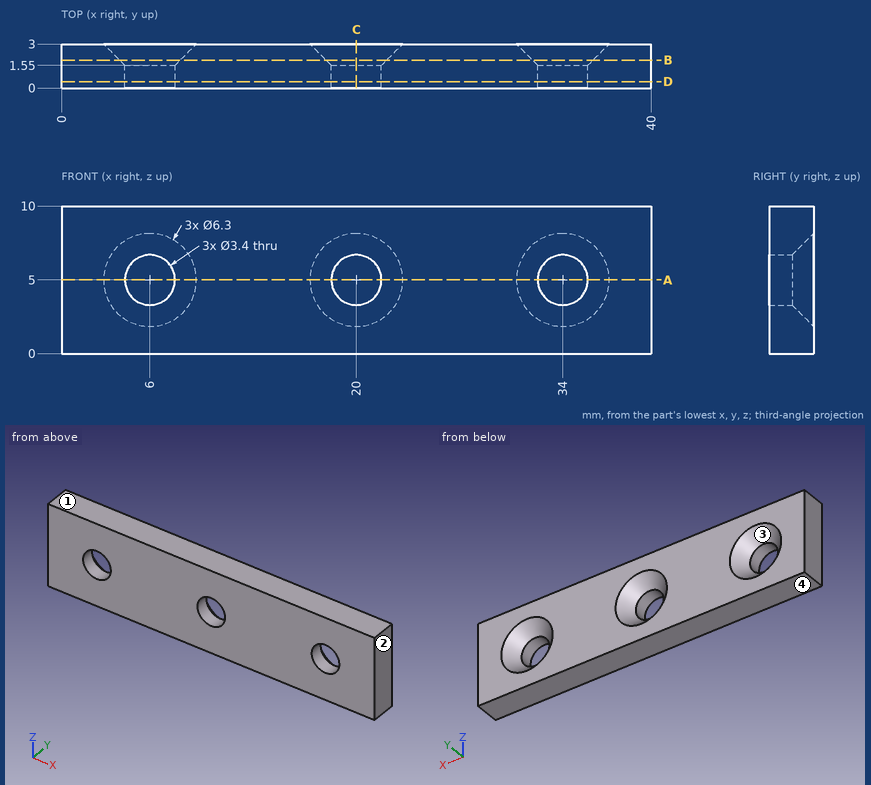
Design review of the part shown in the three views and the two pictorial views. Dimensions are in mm from the part's minimum x, y and z. Give positions to 0.01 mm unless a question says otherwise; leave off trailing zeros. Order: outer loops, then holes, each group sorted by start corner. A loop starts at its lowest first (then second) coordinate and runs counter-clockwise, first axis right, second up. Notation, with made-up numbers: M -37,23 L 10,23 A19 ccw 10,59 Z; hole C -36.75,10.25 d4. An arc over 180 degrees is marked long. Answer in a Markdown table with one row per item. Add a question column.
(1) For pin 1 (4 mm diameter, centred on x = 6, z = 5, fed in from +Y); pin 2 (2.5 mm diameter, centred on x = 34, z = 5, fed in from +Y); pin 3 (3 mm diameter, centred on x = 7.5, z = 5, fed in from +Y), all flat-tipped, find the tip position at first contact; note any pin that passes through.
(2) Consider section D-D on y = 0.45. State the section outline as (x, z) points.
(3) Wall thickness on probe 1 along X at (y, z) = (0.7, 5); probe 2 along Z at (x, y) = (6, 0.8); probe 3 along X at (y, z) = (1.9, 5): over which ranges is each line inside the solid? List them lowest first. Write a range as [from, to].
(4) Mouldability with a two-part tool opening along Z and no side actions: class the marked faces 1, 2, 3 and 4 as +Z half, -Z half, draft (parallel to the pull), parting line (faces both ways), or undercut.
(5) Consider section C-C on x = 20. State the section outline as (y, z) points.
(6) Consider section B-B on y = 1.9. State the section outline as (x, z) points, and give its area (3 significant figures).
(7) Consider section A-A on z = 5. State the section outline as (x, y) points.
Evaluation:
| question | item | result |
|---|---|---|
| 1 | pin 1 | stops at y = 1.85 |
| 1 | pin 2 | passes through |
| 1 | pin 3 | stops at y = 2.85 |
| 2 | outline | M 0,0 L 40,0 L 40,10 L 0,10 Z; hole C 6,5 d3.4; hole C 20,5 d3.4; hole C 34,5 d3.4 |
| 3 | probe 1 | x = [0, 4.3], [7.7, 18.3], [21.7, 32.3], [35.7, 40] |
| 3 | probe 2 | z = [0, 3.3], [6.7, 10] |
| 3 | probe 3 | x = [0, 3.95], [8.05, 17.95], [22.05, 31.95], [36.05, 40] |
| 4 | face 1 | +Z half |
| 4 | face 2 | draft |
| 4 | face 3 | undercut |
| 4 | face 4 | -Z half |
| 5 | outline | M 0,0 L 3,0 L 3,1.85 L 1.55,3.3 L 0,3.3 Z; M 0,6.7 L 1.55,6.7 L 3,8.15 L 3,10 L 0,10 Z |
| 6 | outline | M 0,0 L 40,0 L 40,10 L 0,10 Z; hole C 6,5 d4.1; hole C 20,5 d4.1; hole C 34,5 d4.1 |
| 6 | area | 360 mm^2 |
| 7 | outline | M 0,0 L 4.3,0 L 4.3,1.55 L 2.85,3 L 0,3 Z; M 7.7,0 L 18.3,0 L 18.3,1.55 L 16.85,3 L 9.15,3 L 7.7,1.55 Z; M 21.7,0 L 32.3,0 L 32.3,1.55 L 30.85,3 L 23.15,3 L 21.7,1.55 Z; M 35.7,0 L 40,0 L 40,3 L 37.15,3 L 35.7,1.55 Z |
